Can you work these out from the model? Positions are in its coordinate system, mm. Face numbers are marked on the shaded views. A direction names the side the tool comes from. Round coordinates to 2 decimals unless told otherwise and drop trailing zeros. Order: outer loops, then holes, each group sorted by start corner. A loop starts at its lowest first (then second) coordinate and runs counter-clockwise, first axis right, second up. Notation, with made-up numbers: (-23.75, 64.25) -> (-11.75, 64.25) arc R24 cw to (-11.75, 82.25) -> close; hole circle Ø3 at (26.5, 81.25). An arc over 180 degrees is marked (long way). One line per item, written item: value.
```python
from build123d import *

# Parameters (mm, degrees)
F0_R     = 5.25
F1_DEPTH = 5
F2_R     = 2.75
F3_DEPTH = 15
F4_R     = 2.75
F5_DEPTH = 15
F6_R     = 1.275
F7_DEPTH = 5.001
F8_R     = 2.5


with BuildPart() as f1:
    # F0 (on Top) → F1 (new body)
    with BuildSketch(Plane.XY):
        with BuildLine():
            ThreePointArc((27.8461538462, 8.4807692308), (0, 5), (-27.8461538462, 8.4807692308))
            ThreePointArc((-27.8461538462, 8.4807692308), (-33.4013149384, 8.0618581412), (-37.5777222831, 4.375))
            Line((-37.5777222831, 4.375), (-50.2027222831, -17.4921414456))
            Line((-50.2027222831, -17.4921414456), (-35.0472777169, -26.2421414456))
            Line((-35.0472777169, -26.2421414456), (-29.8445554338, -17.2307621135))
            ThreePointArc((-29.8445554338, -17.2307621135), (0, 0), (29.8445554338, -17.2307621135))
            Line((29.8445554338, -17.2307621135), (35.0472777169, -26.2421414456))
            Line((35.0472777169, -26.2421414456), (50.2027222831, -17.4921414456))
            Line((50.2027222831, -17.4921414456), (37.5777222831, 4.375))
            ThreePointArc((37.5777222831, 4.375), (33.4013149384, 8.0618581412), (27.8461538462, 8.4807692308))
        make_face()
        with Locations((-30, 0)):
            Circle(F0_R, mode=Mode.SUBTRACT)
        with Locations((30, 0)):
            Circle(F0_R, mode=Mode.SUBTRACT)
    extrude(amount=F1_DEPTH)

    # F2 (on face) → F3 (cut)
    with BuildSketch(Plane(origin=(-20.125, -34.8575225023, 0), x_dir=(0.8660254038, -0.5, 0), z_dir=(-0.5, -0.8660254038, 0))):
        with Locations((-25.9807621135, 0)):
            Circle(F2_R)
    extrude(amount=-F3_DEPTH, mode=Mode.SUBTRACT)

    # F4 (on face) → F5 (cut)
    with BuildSketch(Plane(origin=(20.125, -34.8575225023, 0), x_dir=(0.8660254038, 0.5, 0), z_dir=(0.5, -0.8660254038, 0))):
        with Locations((25.9807621135, 0)):
            Circle(F4_R)
    extrude(amount=-F5_DEPTH, mode=Mode.SUBTRACT)

    # F6 (on face) → F7 (cut, through all)
    with BuildSketch(Plane(origin=(0, 0, 0), x_dir=(1, 0, 0), z_dir=(0, 0, -1))):
        with Locations((-46.7876587737, 16.5770779361)):
            Circle(F6_R)
        with Locations((-35.9623412263, 22.8270779361)):
            Circle(F6_R)
        with Locations((35.9623412263, 22.8270779361)):
            Circle(F6_R)
        with Locations((46.7876587737, 16.5770779361)):
            Circle(F6_R)
    extrude(amount=-F7_DEPTH, mode=Mode.SUBTRACT)

    # F8
    f8_edges = [f1.edges().sort_by_distance(p)[0] for p in [
        (-50.202722, -17.492141, 2.5),
        (-35.047278, -26.242141, 2.5),
        (35.047278, -26.242141, 2.5),
        (50.202722, -17.492141, 2.5),
    ]]
    fillet(f8_edges, radius=F8_R)


solid = f1.part
```
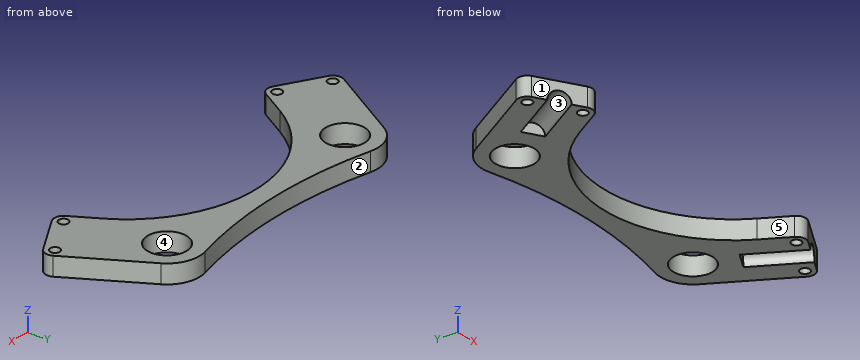
Q1. I want a section at A-A on z = 1.9. List the corners of the cut face in (x, y) for me (3 decimals).
Answers below:
outline: (-48.953, -15.327) arc R2.5 ccw to (-48.038, -18.742) -> (-44.347, -20.873) -> (-36.847, -7.883) -> (-33.403, -9.871) -> (-40.903, -22.861) -> (-37.212, -24.992) arc R2.5 ccw to (-33.797, -24.077) -> (-29.845, -17.231) arc R34.462 cw to (29.845, -17.231) -> (33.797, -24.077) arc R2.5 ccw to (37.212, -24.992) -> (40.903, -22.861) -> (33.403, -9.871) -> (36.847, -7.883) -> (44.347, -20.873) -> (48.038, -18.742) arc R2.5 ccw to (48.953, -15.327) -> (37.578, 4.375) arc R8.75 ccw to (27.846, 8.481) arc R113.125 cw to (-27.846, 8.481) arc R8.75 ccw to (-37.578, 4.375) -> close; hole circle Ø2.55 at (-46.788, -16.577); hole circle Ø2.55 at (-35.962, -22.827); hole circle Ø10.5 at (-30, 0); hole circle Ø10.5 at (30, 0); hole circle Ø2.55 at (35.962, -22.827); hole circle Ø2.55 at (46.788, -16.577)
Q2. Please list where these lines run through material, in increasing order: line 1 along X through (y, z) = (0.5, 1.3); line 2 along X through (y, z) = (-9.5, 1.55); line 3 along X through (y, z) = (-6, 3.8).
Answers below:
line 1: -39.81 to -35.23, -24.77 to 24.77, 35.23 to 39.81
line 2: -45.59 to -38.11, -34.05 to -23.76, 23.76 to 34.05, 38.11 to 45.59
line 3: -43.57 to -19.43, 19.43 to 43.57
Q3. I want a section at B-B on x = -21.5. List the corners of the cut face in (y, z) for me.
Answers below:
outline: (-7.53, 0) -> (7.06, 0) -> (7.06, 5) -> (-7.53, 5) -> close
Q4. I want a section at C-C on x = 13.5. List the corners of the cut face in (y, z) for me, plus the area to 3 significant figures.
Answers below:
outline: (-2.75, 0) -> (5.81, 0) -> (5.81, 5) -> (-2.75, 5) -> close
area: 42.8 mm^2
Q5. On a 3-axis mill with a long thin cutter (end or side, diameter ignored), from which of +Z, -Z, +X, -X, +Y, -Y can I reach the whole of each face in a straight line? I mean the marked faces 4 and 5. Say none if no direction works.
Answers below:
face 4: +Z, -Z
face 5: +Z, -Z, -Y
Q6. Will these pins go through, and if not, where does the flat tip stop? pin 1 Ø1.5 at (y, z) = (3, 3.5) entering from -X; pin 2 Ø1 at (y, z) = (-13.5, 3.5) entering from -X; pin 3 Ø3 at (y, z) = (-9.5, 2.5) entering from +X.
Answers below:
pin 1: x = -38.8
pin 2: x = -48.19
pin 3: x = 46.45
Q7. We'd pull the mould along Y, two halves only. Please class the marked faces 1, 2 and 3: released by +Y, released by -Y, zero draft, split by the parting line, or undercut.
Answers below:
face 1: released by -Y
face 2: released by +Y
face 3: undercut
